The figure shows three views and two pictorial views of one solid part (mm, origin at its lowest corner). Answer the questions. A direction names the side the tool comes from. Coordinates: 2 decimals unless noted, no trailing zeros. Order: outer loops, then holes, each group sorted by start corner. A loop starts at its lowest first (then second) coordinate and runs counter-clockwise, first axis right, second up. Notation, with made-up numbers: M 7,20.25 L 16,20.25 A23 cw 16,37.25 Z; hole C -10.5,41.25 d7. An arc over 180 degrees is marked long. Answer in a Markdown table with one row per item. Add a question column.
Item 1: The part is cut by section B-B (y = 45). Write down the section's boundary in (x, z).
Item 2: The mould has two halves that part along X. Classify the marked faces 4, 5, 6 and 7: released by +X, released by -X, zero draft, split by the parting line, or undercut.
Item 3: The part is cut by section D-D (y = 22). Write down the section's boundary in (x, z), then the cut area to 3 significant figures.
Item 4: Consider line 1 (Z direction, x = 10, y = 37); line 2 (X direction, y = 50, z = 10); line 3 (X direction, y = 12, z = 11.75). Determine where each line is inside the solid, lowest interval first. Write a range as from..to.
Item 5: Which of the six approach directions +Z, -Z, +X, -X, +Y, -Y give full straight-line access (tool end or side, diameter ignored) to the marked faces 1, 2 and 3?
Item 6: Flat-ended cylindrical pins translate along their axes: pin 1 Ø9 at (x, z) = (10, 10) entering from +Y; pin 2 Ø11 at (y, z) = (61, 15) entering from -X; pin 3 Ø8 at (y, z) = (60.5, 9) entering from +X. Find the tip coordinate at first contact, or state that the pin passes through.
Item 7: The part is cut by section C-C (x = 40.5). Write down the section's boundary in (y, z), then the cut area to 3 significant figures.
Item 8: The part is cut by section A-A (z = 10). Write down the section's boundary in (x, y), then the cut area to 3 significant figures.
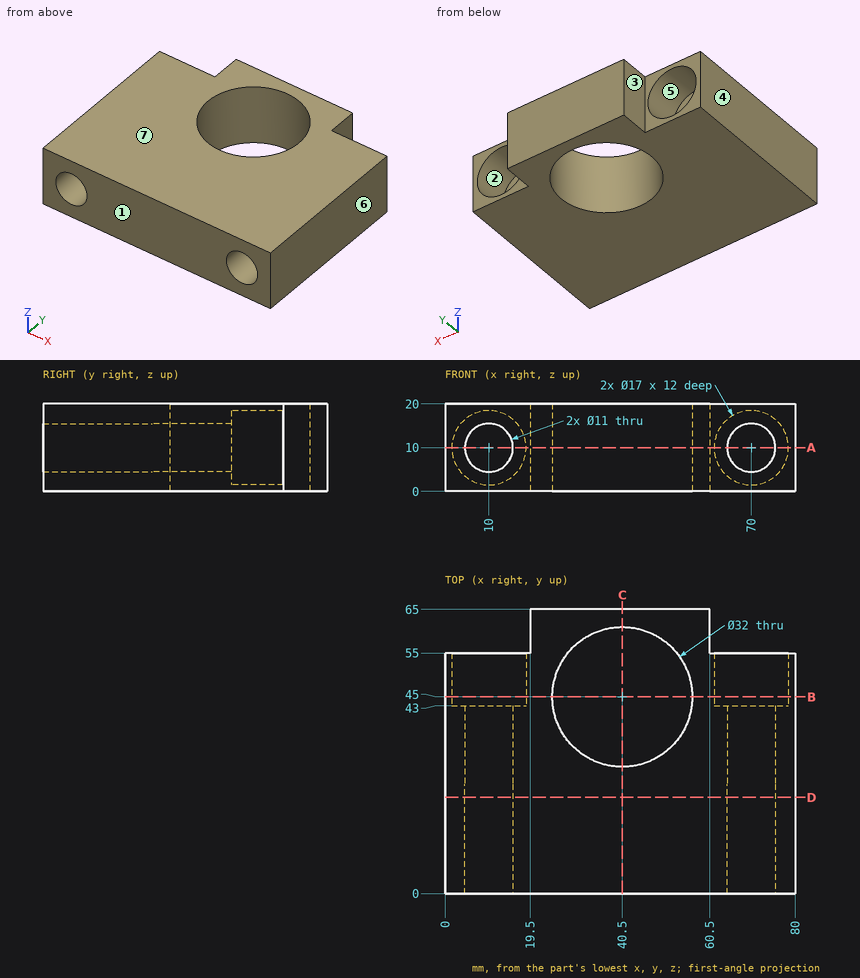
Reply:
| question | item | result |
|---|---|---|
| 1 | outline | M 0,0 L 24.5,0 L 24.5,20 L 0,20 Z; M 56.5,0 L 80,0 L 80,20 L 56.5,20 Z; hole C 10,10 d17; hole C 70,10 d17 |
| 2 | face 4 | released by -X |
| 2 | face 5 | undercut |
| 2 | face 6 | released by +X |
| 2 | face 7 | zero draft |
| 3 | outline | M 0,0 L 80,0 L 80,20 L 0,20 Z; hole C 10,10 d11; hole C 70,10 d11 |
| 3 | area | 1,410 mm2 |
| 4 | line 1 | z = 0..4.5, 15.5..20 |
| 4 | line 2 | x = 0..1.5, 18.5..25.3, 55.7..61.5, 78.5..80 |
| 4 | line 3 | x = 0..4.79, 15.21..64.79, 75.21..80 |
| 5 | face 1 | +Z, -Z, +X, -X, -Y |
| 5 | face 2 | +Y |
| 5 | face 3 | +Z, -Z, -X, +Y |
| 6 | pin 1 | passes through |
| 6 | pin 2 | stops at x = 19.5 |
| 6 | pin 3 | stops at x = 60.5 |
| 7 | outline | M 0,0 L 29,0 L 29,20 L 0,20 Z; M 61,0 L 65,0 L 65,20 L 61,20 Z |
| 7 | area | 660 mm2 |
| 8 | outline | M 0,0 L 4.5,0 L 4.5,43 L 1.5,43 L 1.5,55 L 0,55 Z; M 15.5,0 L 64.5,0 L 64.5,43 L 61.5,43 L 61.5,55 L 60.5,55 L 60.5,65 L 19.5,65 L 19.5,55 L 18.5,55 L 18.5,43 L 15.5,43 Z; M 75.5,0 L 80,0 L 80,55 L 78.5,55 L 78.5,43 L 75.5,43 Z; hole C 40.5,45 d32 |
| 8 | area | 2,650 mm2 |
